CAD build for the part. Positions are in the model's coordinates, mm. A direction names the side the tool comes from. Give positions to 0.01 mm unless a question says otherwise; leave off trailing zeros. Loops run counter-clockwise (first coordinate to the right, second up) from the corner with the lowest first, then second, coordinate; pieces in that order, holes last. Notation, with made-up numbers: (85.5, 1.25) -> (104.5, 1.25) arc R9 ccw to (104.5, 5.25) -> close; hole circle Ø1 at (31, 9). An arc over 180 degrees is marked (long way). Write each question's results on one line, items separated by ' | '. Start each with the question number.
Autodesk Inventor part; units mm, degrees
ref_plane "YZ Plane" through (0, 0, 0) normal (1, 0, 0) x (0, 1, 0)
ref_plane "XZ Plane" through (0, 0, 0) normal (0, 1, 0) x (-1, 0, 0)
ref_plane "XY Plane" through (0, 0, 0) normal (0, 0, 1) x (1, 0, 0)
sketch "Sketch1" plane through (0, 0, 0) normal (0, 0, 1) x (1, 0, 0)
  arc A0 (-167.2585, -83.0448) -> (135.7751, 278.0965) centre (-230.9374, 278.0965) ccw
  line L0 (135.7751, 278.0965) -> (135.7751, 439.2052)
  line L1 (132.6001, 439.2052) -> (135.7751, 439.2052)
  line L2 (132.6001, 439.2052) -> (132.6001, 278.0965)
  arc A1 (-167.8098, -79.9181) -> (132.6001, 278.0965) centre (-230.9374, 278.0965) ccw
  line L3 (-167.8098, -79.9181) -> (-386.5124, -118.4812)
  line L4 (-386.5124, -121.7052) -> (-386.5124, -118.4812)
  line L5 (-386.5124, -121.7052) -> (-167.2585, -83.0448)
  point P0 (0, 0)
extrude "Extrusion1" add sketch "Sketch1" along normal blind 117.475
hole "Hole1" at (135.7751, 426.5052, 109.5375) direction (-1, 0, 0) diameter 6.731 depth 25.4 tip angle 118
pattern_linear "Rectangular Pattern1" count 2 spacing 133.35 along (0, -1, 0) of "Hole1"
hole "Hole2" at (-374.0054, -119.4999, 109.5375) direction (-0.1736, 0.9848, 0) diameter 6.731 depth 25.4 tip angle 118
pattern_linear "Rectangular Pattern2" count 2 spacing 190.5 along (0.9848, 0.1736, 0) of "Hole2"
pattern_linear "Rectangular Pattern3" count 2 spacing 68.2625 along (0, 0, -1) of "Hole1"
properties part number "GE-12071-02"
Q1. Wall check: L1, parallel to X at y = 305.5, z = 99; L2, parallel to Y at x = -9.5, z = 66.5; L3, parallel to Y at x = -50, z = 17.5. Give the ranges that are in metal, low to high.
Q2. Saw through at B-B, the plane y = 226. List the corners of the cut face in (x, z) (3 decimals), then the cut area to 3 significant figures.
Q3. Saw through at C-C, the plane x = 96. List the corners of the cut face in (y, z) (3 decimals).
Q4. Saw through at A-A, the plane z = 76.5. List the corners of the cut face in (x, y).
Q5. Which spindle directions (+Z, -Z, +X, -X, +Y, -Y) get a long thin tool onto all of the face, cutting with end or side? Do faces 1 (the face through (52.271, 45.135, 57.915)), 2 (the face through (132.6, 360, 58)). Say none if no direction does.
Q6. Drop flat-ended pins along their axis: pin 1 (8 mm diameter, centred on y = 232, z = 75.5, fed in from +X); pin 2 (2 mm diameter, centred on x = 11, z = 15, fed in from -Y); pin 3 (7.5 mm diameter, centred on y = 426.51, z = 41.28, fed in from -X); pin 4 (9 mm diameter, centred on y = 293.16, z = 109.54, fed in from +X). Give the stop position or say it passes through.
Answer block:
1) L1: x = 132.6 to 135.78 | L2: y = -14.21 to -10.22 | L3: y = -40.87 to -37.21
2) outline: (128.848, 0) -> (132.056, 0) -> (132.056, 117.475) -> (128.848, 117.475) -> close | area: 377 mm2
3) outline: (111.994, 0) -> (119.126, 0) -> (119.126, 117.475) -> (111.994, 117.475) -> close
4) outline: (-386.51, -121.71) -> (-167.26, -83.04) arc R366.71 ccw to (135.78, 278.1) -> (135.78, 439.21) -> (132.6, 439.21) -> (132.6, 278.1) arc R363.54 cw to (-167.81, -79.92) -> (-386.51, -118.48) -> close
5) face 1: +Z, -Z, +X, -Y | face 2: +Z, -Z, -X, +Y
6) pin 1: stops at x = 133.35 | pin 2: stops at y = 1.64 | pin 3: stops at x = 132.6 | pin 4: stops at x = 135.78
